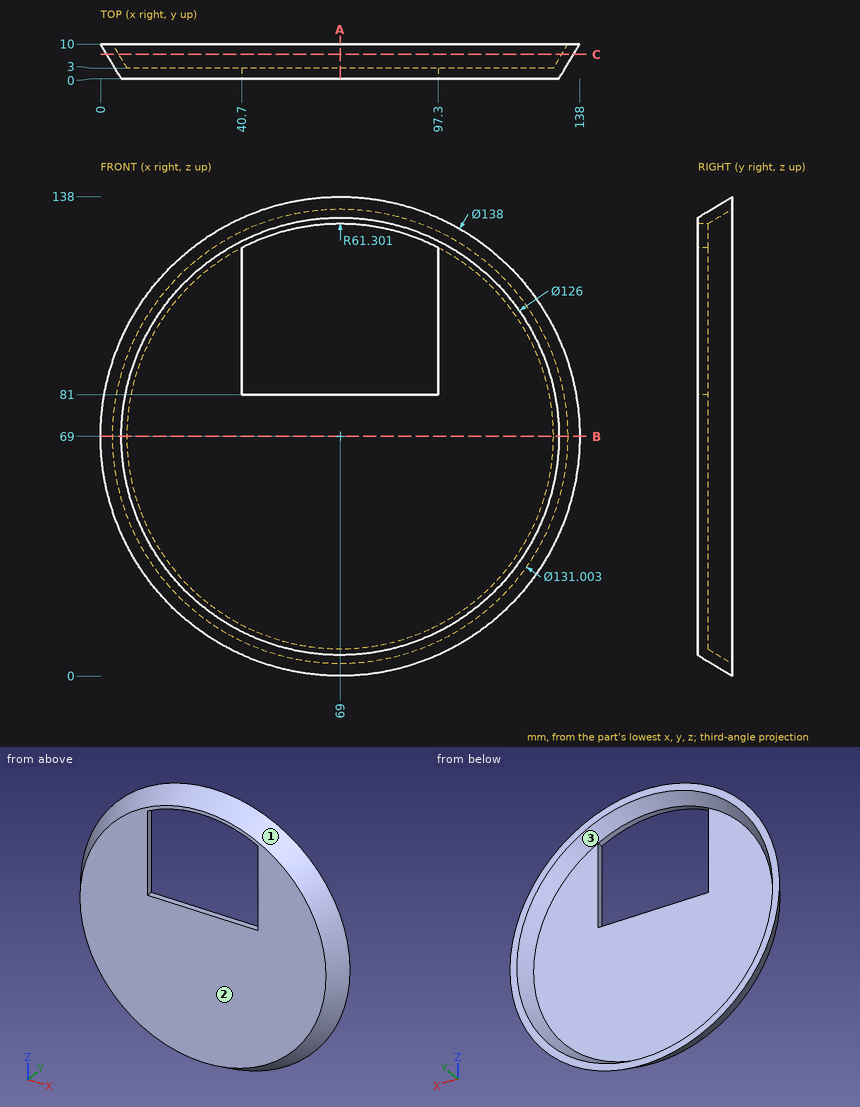
Study the drawing (mm; zero at the part's minimum x, y, z) and answer. Give positions to 0.01 mm unless a question says otherwise; leave off trailing zeros. Loops run counter-clockwise (first coordinate to the right, second up) from the corner with the lowest first, then second, coordinate; pieces in that order, holes last. Notation, with made-up numbers: M 49,-26.5 L 86,-26.5 A31 cw 86,10.5 Z; hole C 88,17.5 d9. An arc over 180 degrees is marked long. Answer as CSV lines item,"result".
Item 1: The part is cut by section C-C (y = 7). Give the vertices of the cut face in (x, z).
Values follow:
outline,"C 69,69 d134.4; hole C 69,69 d127.4"
Item 2: The mould has two halves that part along X. Classify the marked faces 1, 2 and 3: released by +X, released by -X, zero draft, split by the parting line, or undercut.
Values follow:
face 1,"split by the parting line"
face 2,"zero draft"
face 3,"undercut"
Item 3: Given pin 1 Ø2 at (x, z) = (75, 78) entering from +Y; pin 2 Ø2.5 at (x, y) = (64.5, 1) entering from +Z; pin 3 Ø0.9 at (y, z) = (1, 98.5) entering from +X; pin 4 Ø1.5 at (x, z) = (123.5, 100.5) entering from -Y, each flat-ended and moving along its own axis, determine where each tip first touches the part or whether it passes through.
Values follow:
pin 1,"stops at y = 3"
pin 2,"stops at z = 133.2"
pin 3,"stops at x = 125.73"
pin 4,"stops at y = 0"
Item 4: Straight lines are drawn through the part: line 1 along Y through (x, z) = (107, 97); line 2 along Z through (x, y) = (88, 1) (1 decimal); line 3 along X through (y, z) = (8, 24) (1 decimal). For each, find the intervals that lie inside material, in ascending order. Write a range as [from, to].
Values follow:
line 1,"y = [0, 3]"
line 2,"z = [8.3, 81], [127.3, 129.7]"
line 3,"x = [18.3, 23.1], [114.9, 119.7]"
Item 5: The part is cut by section B-B (z = 69). Give the vertices of the cut face in (x, y).
Values follow:
outline,"M 0,10 L 6,0 L 132,0 L 138,10 L 134.5,10 L 130.3,3 L 7.7,3 L 3.5,10 Z"
Item 6: The part is cut by section A-A (x = 69). Give the vertices of the cut face in (y, z).
Values follow:
outline,"M 0,6 L 10,0 L 10,3.5 L 3,7.7 L 3,81 L 0,81 Z; M 0,130.3 L 3,130.3 L 10,134.5 L 10,138 L 0,132 Z"
